Read the model definition and answer for the solid it produces. Units are mm, in the model's axes. A direction names the side the tool comes from. Round coordinates to 2 decimals unless told otherwise and drop trailing zeros. Write each loop counter-clockwise with the first axis right and the second up, starting at its lowest first coordinate (ties: lowest second). Pieces come first, ordered by that corner, then holes. Notation, with made-up numbers: (-14.5, -11) -> (9.5, -11) arc R22 ccw to (9.5, 3) -> close; hole circle Ø9 at (80.25, 33). An arc over 180 degrees is marked (long way). Return JSON: item names as keys, results as strings.
from build123d import *

# Parameters (mm, degrees)
SKETCH1_R           = 1.5
BOSS_EXTRUDE1_DEPTH = 20
SKETCH2_R           = 1.5
BOSS_EXTRUDE2_DEPTH = 1


with BuildPart() as part:
    # Sketch1 → Boss-Extrude1 (new, symmetric)
    with BuildSketch(Plane(origin=(0, 0, 0), x_dir=(1, 0, 0), z_dir=(0, 1, 0))):
        with Locations(Location((0, 0, 0), (0, 0, 270))):
            Circle(SKETCH1_R)
    extrude(amount=BOSS_EXTRUDE1_DEPTH, both=True)

    # Sketch2 → Boss-Extrude2 (add, symmetric)
    with BuildSketch(Plane(origin=(0, 0, 0), x_dir=(1, 0, 0), z_dir=(0, 1, 0))):
        with BuildLine():
            Line((-50.941176471, 2.999423243), (0.039215686, 1.999615496))
            ThreePointArc((0.039215686, 1.999615496), (2, 0), (0.039215686, -1.999615496))
            Line((0.039215686, -1.999615496), (-50.941176471, -2.999423243))
            ThreePointArc((-50.941176471, -2.999423243), (-54, 0), (-50.941176471, 2.999423243))
        make_face()
        with Locations(Location((-51, 0, 0), (0, 0, 270))):
            Circle(SKETCH2_R, mode=Mode.SUBTRACT)
    extrude(amount=BOSS_EXTRUDE2_DEPTH, both=True)


solid = part.part
Item 1: Straight lines are drawn through the part: L1, parallel to X at y = 0.2, z = 0; L2, parallel to Y at x = -48.5, z = 2.1; L3, parallel to X at y = 14.5, z = 1.2. For each, find the intervals that lie inside material, in ascending order. Write a range as [from, to].
Worked answers:
{"L1": "x = [-54, -52.5], [-49.5, 2]", "L2": "y = [-1, 1]", "L3": "x = [-0.9, 0.9]"}
Item 2: For a pull along X with two mould halves and no side action, classify faces 4 (the cylindrical face through (-52.464, -0.014, -0.325)), 5 (the cylindrical face through (2, 0, 0)), 6 (the flat face through (0, 20, 0)) as released by +X, released by -X, zero draft, split by the parting line, or undercut.
Worked answers:
{"face 4": "undercut", "face 5": "released by +X", "face 6": "zero draft"}
Item 3: Section C-C (x = -19.5) is taken. Give the vertices of the cut face in (y, z).
Worked answers:
{"outline": "(-1, -2.38) -> (1, -2.38) -> (1, 2.38) -> (-1, 2.38) -> close"}
Item 4: Flat-ended cylindrical pins translate along their axes: pin 1 (2 mm diameter, centred on x = -28, z = -0.5, fed in from +Y); pin 2 (5 mm diameter, centred on x = -24, y = -3, fed in from +Z); pin 3 (1 mm diameter, centred on x = -29, z = 1.5, fed in from -Y). Find the tip coordinate at first contact, or state that the pin passes through.
Worked answers:
{"pin 1": "stops at y = 1", "pin 2": "stops at z = 2.5", "pin 3": "stops at y = -1"}
Item 5: Section D-D (x = -5.5) is taken. Give the vertices of the cut face in (y, z).
Worked answers:
{"outline": "(-1, -2.11) -> (1, -2.11) -> (1, 2.11) -> (-1, 2.11) -> close"}
Item 6: Section A-A (z = 0) is taken. Give the vertices of the cut face in (x, y), then the cut area to 3 significant figures.
Worked answers:
{"outline": "(-54, -1) -> (-52.5, -1) -> (-52.5, 1) -> (-54, 1) -> close; (-49.5, -1) -> (-1.5, -1) -> (-1.5, -20) -> (1.5, -20) -> (1.5, -1) -> (2, -1) -> (2, 1) -> (1.5, 1) -> (1.5, 20) -> (-1.5, 20) -> (-1.5, 1) -> (-49.5, 1) -> close", "area": "220 mm2"}
Item 7: Section B-B (y = -5) is taken. Give the vertices of the cut face in (x, z).
Worked answers:
{"outline": "circle Ø3 at (0, 0)"}
Item 8: A tool of negligible diameter and unlimited length cuts with its end or side. For faces 1 (the cylindrical face through (0.45, -10.37, 1.43)), 2 (the cylindrical face through (0.45, 10.63, 1.43)), 3 (the flat face through (0, -20, 0)), from which of +Z, -Z, +X, -X, +Y, -Y can it reach the whole face along a straight path? Write none if from no direction.
Worked answers:
{"face 1": "-Y", "face 2": "+Y", "face 3": "+Z, -Z, +X, -X, -Y"}
